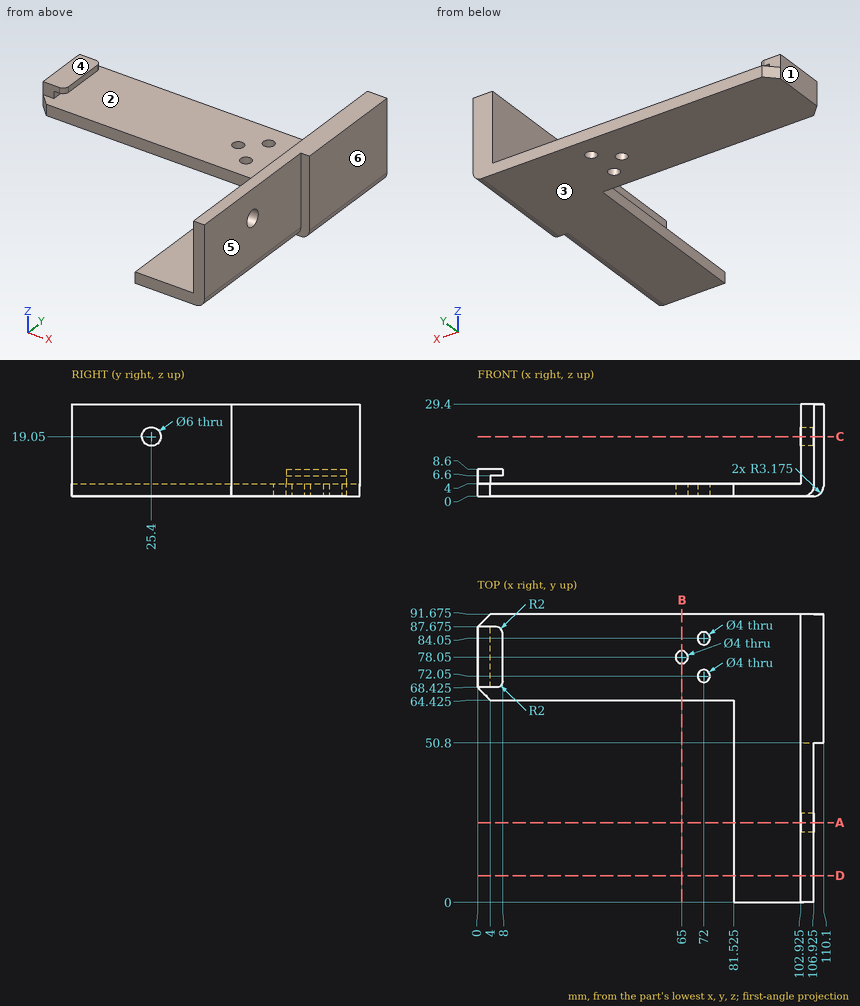
Geometry check sheet. Reference: drawing and pictorial views, mm from the part's lowest x, y, z. A direction names the side the tool comes from. Give positions to 0.01 mm unless a question says otherwise; leave off trailing zeros. Order: outer loops, then holes, each group sorted by start corner. A loop starts at its lowest first (then second) coordinate and runs counter-clockwise, first axis right, second up. Notation, with made-up numbers: M 2,-12 L 47,-12 A16 cw 47,11 Z; hole C 33,-12 d7. An arc over 180 degrees is marked long. Answer in a Markdown table with one row per item. Add a question column.
Q1. Sectioned sample at A-A, the plane y = 25.4. Record the boundary of the cut face in (x, z) (3 decimals).
Q2. Access from +Z, -Z, +X, -X, +Y, -Y to the whole of each face (thin tool, end or side, straight path). Record for the marked faces 4, 5 and 6.
Q3. Sectioned sample at D-D, the plane y = 8.5. Record the boundary of the cut face in (x, z) (3 decimals), and give its area (3 significant figures).
Q4. Sectioned sample at B-B, the plane x = 65. Record the boundary of the cut face in (y, z) (3 decimals), and give its area (3 significant figures).
Q5. Sectioned sample at C-C, the plane z = 19.05. Record the boundary of the cut face in (x, y) (3 decimals).
Q6. Release check for a two-part mould opening along X. For the marked faces 1, 2 and 3 record: released by +X, released by -X, zero draft, split by the parting line, or undercut.
Q7. Thickness scan on L1, parallel to Y at x = 72, z = 1.65 (3 decimals); L2, parallel to Y at x = 104.9, z = 19.05 (3 decimals); L3, parallel to X at y = 40, z = 20 (3 decimals). Record the ranges inside material, lowest first.
Q8. Gauge pin test, flat ends, axial feed: pin 1 Ø1.2 at (y, z) = (39, 3) entering from -X (3 decimals); pin 2 Ø2.5 at (x, y) = (4.5, 75) entering from +Z; pin 3 Ø13 at (y, z) = (28, 11) entering from +X (3 decimals); pin 4 Ø2.5 at (x, y) = (65, 78.05) entering from +Z. Record the tip position at first contact, or that the pin passes through.
Verdict:
| question | item | result |
|---|---|---|
| 1 | outline | M 81.525,0 L 103.75,0 A3.175 ccw 106.925,3.175 L 106.925,16.05 L 102.925,16.05 L 102.925,4 L 81.525,4 Z; M 102.925,22.05 L 106.925,22.05 L 106.925,29.4 L 102.925,29.4 Z |
| 2 | face 4 | +Z, -X, +Y, -Y |
| 2 | face 5 | +Z, -Z, +X, -Y |
| 2 | face 6 | +Z, -Z, +X, +Y, -Y |
| 3 | outline | M 81.525,0 L 103.75,0 A3.175 ccw 106.925,3.175 L 106.925,29.4 L 102.925,29.4 L 102.925,4 L 81.525,4 Z |
| 3 | area | 201 mm² |
| 4 | outline | M 64.425,0 L 76.05,0 L 76.05,4 L 64.425,4 Z; M 80.05,0 L 91.675,0 L 91.675,4 L 80.05,4 Z |
| 4 | area | 93.0 mm² |
| 5 | outline | M 102.925,0 L 106.925,0 L 106.925,22.4 L 102.925,22.4 Z; M 102.925,28.4 L 106.925,28.4 L 106.925,50.8 L 110.1,50.8 L 110.1,91.675 L 102.925,91.675 Z |
| 6 | face 1 | released by -X |
| 6 | face 2 | undercut |
| 6 | face 3 | zero draft |
| 7 | L1 | 64.425 to 70.05, 74.05 to 82.05, 86.05 to 91.675 |
| 7 | L2 | 0 to 22.4, 28.4 to 91.675 |
| 7 | L3 | 102.925 to 106.925 |
| 8 | pin 1 | x = 81.525 |
| 8 | pin 2 | z = 8.6 |
| 8 | pin 3 | x = 106.925 |
| 8 | pin 4 | through |
